Print and shaded views of the part. All mm, measured from the part's lowest x, y and z. A direction names the side the tool comes from. Round coordinates to 2 decimals unless told otherwise and drop trailing zeros. Loops run counter-clockwise (first coordinate to the right, second up) from the corner with the lowest first, then second, coordinate; pieces in that order, holes last. Notation, with made-up numbers: (18.25, 7) - (47.25, 7) arc R12 cw to (47.25, 30) - close; hole circle Ø10 at (41.5, 37). An arc over 180 degrees is marked (long way). Use one line per item in the form item = value.
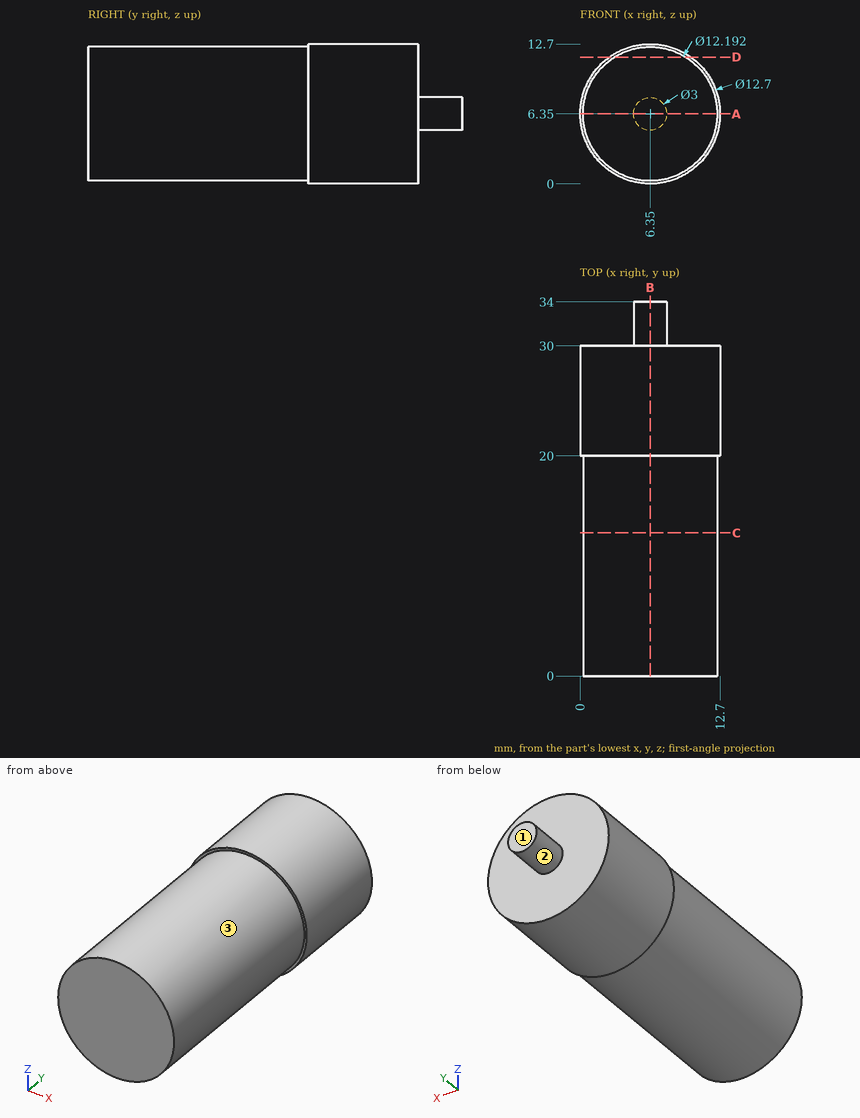
1) Slice it at C-C (y = 13). Write the cut outline in (x, z), plus the area to 3 significant figures.
Report:
outline = circle Ø12.19 at (6.35, 6.35)
area = 117 mm^2
2) Tool access for the marked faces 1, 2 and 3: list every direction of +Z, -Z, +X, -X, +Y, -Y with a clear straight run to the whole face (end or side of a thin tool).
Report:
face_1 = +Z, -Z, +X, -X, +Y
face_2 = +Y
face_3 = -Y
3) Slice it at A-A (z = 6.35). Write the cut outline in (x, y), plus the area to 3 significant figures.
Report:
outline = (0, 20) - (0.25, 20) - (0.25, 0) - (12.45, 0) - (12.45, 20) - (12.7, 20) - (12.7, 30) - (7.85, 30) - (7.85, 34) - (4.85, 34) - (4.85, 30) - (0, 30) - close
area = 383 mm^2
4) Flat gauge pins, fed straight in: pin 1 (1.5 mm diameter, centred on y = 11.5, z = 8.5, fed in from -X); pin 2 (1.5 mm diameter, centred on x = 2, z = 9, fed in from +Y); pin 3 (6 mm diameter, centred on y = 6, z = 6.5, fed in from +X). Where does each tip first touch, or does it go through?
Report:
pin_1 = 0.42
pin_2 = 30
pin_3 = 12.45
5) Slice it at B-B (x = 6.35). Write the cut outline in (y, z).
Report:
outline = (0, 0.25) - (20, 0.25) - (20, 0) - (30, 0) - (30, 4.85) - (34, 4.85) - (34, 7.85) - (30, 7.85) - (30, 12.7) - (20, 12.7) - (20, 12.45) - (0, 12.45) - close
6) Drill centre lines: probe 1 along Y at (x, z) = (0.75, 6.5); probe 2 along Y at (x, z) = (0.5, 4); probe 3 along Z at (x, y) = (10, 27). Where is each one in solid material? Low to high.
Report:
probe_1 = 0 to 30
probe_2 = 20 to 30
probe_3 = 1.15 to 11.55
7) Slice it at D-D (z = 11.5). Write the cut outline in (x, y).
Report:
outline = (2.64, 20) - (3.09, 20) - (3.09, 0) - (9.61, 0) - (9.61, 20) - (10.06, 20) - (10.06, 30) - (2.64, 30) - close
